The listing builds one solid part. Answer for the finished solid, in the listing's coordinates (mm). Give positions to 0.01 mm unless a question says otherwise; leave off trailing zeros. Order: outer loops, then holes, each group sorted by start corner. A loop starts at its lowest first (then second) coordinate and runs counter-clockwise, first axis right, second up. Notation, with made-up numbers: (68, -36) - (115, -36) arc R38 cw to (115, 3) - close; hole circle Ø9 at (-22.75, 49). An arc over 180 degrees is marked (long way). Answer as a JSON object with one key per item and string values. Group by question number.
Q1. A cutting plane is placed at C-C, the plane z = -31.5. Give the vertices of the cut face in (x, y).
Q2. A cutting plane is placed at B-B, the plane x = 26. Give the vertices of the cut face in (y, z), and give its area (3 significant figures).
Q3. Given pin 1 (1.5 mm diameter, centred on x = 19.5, y = -2, fed in from +Z), flat-ended and moving along its own axis, determine where the tip first touches the part or whether it passes through.
Q4. Consider line 1 (Z direction, x = 3, y = -1.1); line 2 (Z direction, x = 9, y = -0.75); line 3 (X direction, y = -0.45, z = -0.5). Determine where each line is inside the solid, lowest interval first.
Q5. A cutting plane is placed at A-A, the plane y = -2.4. Count the separate pieces of the cut face and the enclosed holes in it, and give its area (3 significant figures).
from build123d import *

# Parameters (mm, degrees)
SKETCH_1_R             = 4
SKETCH_1_R_2           = 2
SM_BASE_FLANGE_1_DEPTH = 3


# Sheet-metal steps are written as plain solids
with BuildPart() as part:
    # Sketch 1 → 基体-法兰1 (new body)
    with BuildSketch(Plane(origin=(0, 0, 0), x_dir=(1, 0, 0), z_dir=(0, 1, 0))):
        with BuildLine():
            Line((21.982392954, 200.88), (29.975990392, 1.2))
            ThreePointArc((29.975990392, 1.2), (0, -30), (-29.975990392, 1.2))
            Line((-29.975990392, 1.2), (-21.982392954, 200.88))
            ThreePointArc((-21.982392954, 200.88), (0, 222), (21.982392954, 200.88))
        make_face()
        with Locations(Location((0, 0, 0), (0, 0, 270))):
            Circle(SKETCH_1_R, mode=Mode.SUBTRACT)
        with Locations(Location((0, 200, 0), (0, 0, 270))):
            Circle(SKETCH_1_R, mode=Mode.SUBTRACT)
        with Locations(Location((10, 120, 0), (0, 0, 270))):
            Circle(SKETCH_1_R_2, mode=Mode.SUBTRACT)
        with Locations(Location((-10, 120, 0), (0, 0, 270))):
            Circle(SKETCH_1_R_2, mode=Mode.SUBTRACT)
        with Locations(Location((10, 40, 0), (0, 0, 270))):
            Circle(SKETCH_1_R_2, mode=Mode.SUBTRACT)
        with Locations(Location((-10, 40, 0), (0, 0, 270))):
            Circle(SKETCH_1_R_2, mode=Mode.SUBTRACT)
        with Locations(Location((0, 15, 0), (0, 0, 270))):
            Circle(SKETCH_1_R_2, mode=Mode.SUBTRACT)
        with Locations(Location((15, 0, 0), (0, 0, 270))):
            Circle(SKETCH_1_R_2, mode=Mode.SUBTRACT)
        with Locations(Location((0, -15, 0), (0, 0, 270))):
            Circle(SKETCH_1_R_2, mode=Mode.SUBTRACT)
        with Locations(Location((-15, 0, 0), (0, 0, 270))):
            Circle(SKETCH_1_R_2, mode=Mode.SUBTRACT)
        with Locations(Location((-13.693032158, 200, 0), (0, 0, 270))):
            Circle(SKETCH_1_R_2, mode=Mode.SUBTRACT)
        with Locations(Location((13.693032158, 200, 0), (0, 0, 90))):
            Circle(SKETCH_1_R_2, mode=Mode.SUBTRACT)
    extrude(amount=-SM_BASE_FLANGE_1_DEPTH)


solid = part.part
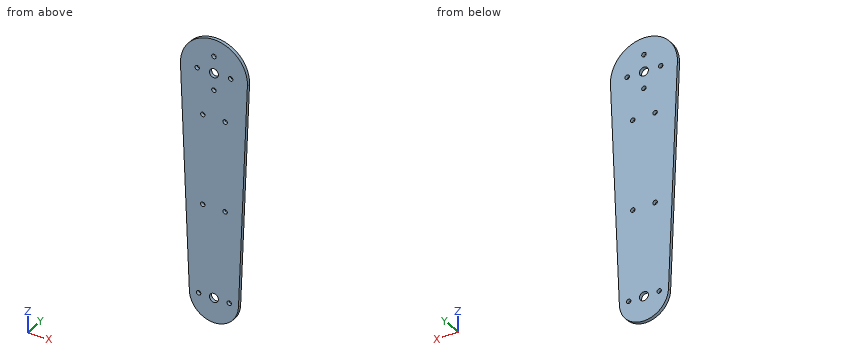
Reply:
{
 "1": {"outline": "(-28.76, -3) - (28.76, -3) - (28.76, 0) - (-28.76, 0) - close"},
 "2": {"outline": "(-3, -100.52) - (0, -100.52) - (0, 14.97) - (-3, 14.97) - close", "area": "346 mm^2"},
 "3": {"pin 1": "stops at z = 23.42"},
 "4": {"line 1": "z = -221.79 to -202.65, -197.35 to -2.65, 2.65 to 29.85", "line 2": "z = -220.07 to -121.73, -118.27 to -41.73, -38.27 to 28.62", "line 3": "x = -30 to -16.94, -13.06 to -3.97, 3.97 to 13.06, 16.94 to 30"},
 "5": {"separate pieces": "1", "enclosed holes": "12", "area": "12,400 mm^2"}
}
